Geometry: final body of the model. Coordinates: model frame, mm. Face numbers are marked on the shaded views. A direction names the side the tool comes from. Round coordinates to 2 decimals unless told otherwise and drop trailing zeros. Loops run counter-clockwise (first coordinate to the right, second up) from the corner with the lowest first, then second, coordinate; pieces in that order, holes last. Notation, with made-up numbers: (85, 21.25) - (115, 21.25) arc R19 ccw to (115, 27.25) - close; hole circle Ø6 at (-3.75, 61.5). An arc over 180 degrees is marked (long way). Use CSV: the item, a comma, the result in double quotes.
from build123d import *

# Parameters (mm, degrees)
TROU_TARAUD_M2_5X0_451_D           = 2.05
TROU_TARAUD_M2_5X0_451_DEPTH       = 7.25
TROU_TARAUD_M2_5X0_451_CSINK_D     = 2.55
TROU_TARAUD_M2_5X0_451_CSINK_ANGLE = 90
TROU_TARAUD_M2_5X0_451_TIP         = 0.615882135


with BuildPart() as part:
    # Esquisse1 → Révolution1 (revolve)
    with BuildSketch(Plane.XY):
        Polygon((0, 16), (58, 16), (58, 2), (71, 2), (71, 0), (-13, 0), (-13, 1.5), (-3, 1.5), (-3, 6.5), (0, 6.5), align=None)
    revolve(axis=Axis((-42.470383275, 0, 0), (1, 0, 0)))

    # Trou taraudé M2.5x0.451
    with Locations(Plane.ZY):
        with Locations((0, 9.5), (-8.227241336, -4.75), (8.227241336, -4.75), (0, -9.5)):
            CounterSinkHole(TROU_TARAUD_M2_5X0_451_D / 2, TROU_TARAUD_M2_5X0_451_CSINK_D / 2, depth=TROU_TARAUD_M2_5X0_451_DEPTH, counter_sink_angle=TROU_TARAUD_M2_5X0_451_CSINK_ANGLE)
            with Locations((0, 0, -(TROU_TARAUD_M2_5X0_451_DEPTH + TROU_TARAUD_M2_5X0_451_TIP / 2))):  # 118° drill point
                Cone(0, TROU_TARAUD_M2_5X0_451_D / 2, TROU_TARAUD_M2_5X0_451_TIP, mode=Mode.SUBTRACT)


solid = part.part
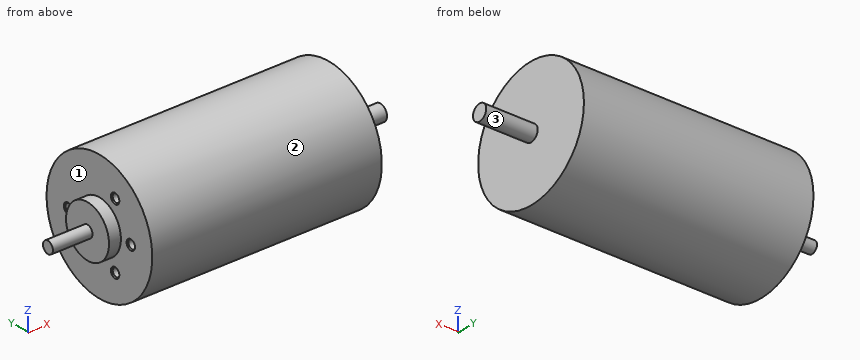
Item 1: Material intervals for line 1 (Z direction, x = 2.5, y = -4.75); line 2 (X direction, y = 6.5, z = -11); line 3 (Z direction, x = 3, y = -4), sorted ascending.
Final values:
line 1,"z = -15.28 to -9.25, -7.2 to 7.2, 9.25 to 15.28"
line 2,"x = 0 to 58"
line 3,"z = -15.49 to -8.93, -7.53 to 7.53, 8.93 to 15.49"
Item 2: Pin query (flat end, axial travel): P1, Ø1.2, axis at y = -4.75, z = -8.23, coming from the +X side; P2, Ø4, axis at x = 36.5, z = 2.5, coming from the +Y side; P3, Ø5, axis at x = 56.5, z = 3, coming from the -Y side. Return the tip coordinate at first contact, or that it passes through.
Final values:
P1,"stops at x = 58"
P2,"stops at y = 15.99"
P3,"stops at y = -15.99"
Item 3: Section D-D on x = 64.5. Return the cut outline in (y, z).
Final values:
outline,"circle Ø4 at (0, 0)"
Item 4: Section A-A on y = 0. Return the cut outline in (x, z).
Final values:
outline,"(-13, -1.5) - (-3, -1.5) - (-3, -6.5) - (0, -6.5) - (0, -16) - (58, -16) - (58, -2) - (71, -2) - (71, 2) - (58, 2) - (58, 16) - (0, 16) - (0, 6.5) - (-3, 6.5) - (-3, 1.5) - (-13, 1.5) - close"
Item 5: Section C-C on x = 47.5. Return the cut outline in (y, z), plus the area to 3 significant figures.
Final values:
outline,"circle Ø32 at (0, 0)"
area,"804 mm²"
Item 6: Section B-B on z = -5. Return the cut outline in (x, y), plus the area to 3 significant figures.
Final values:
outline,"(-3, -4.15) - (0, -4.15) - (0, -15.2) - (58, -15.2) - (58, 15.2) - (0, 15.2) - (0, 4.15) - (-3, 4.15) - close"
area,"1,790 mm²"
Item 7: Reachability of the marked faces 1, 2 and 3 from +Z, -Z, +X, -X, +Y, -Y: full face, straight path, thin tool, end or side. Return the list, or none.
Final values:
face 1,"-X"
face 2,"+X, -X"
face 3,"+X"
